Read the model definition and answer for the solid it produces. Units are mm, in the model's axes. A direction names the side the tool comes from. Round coordinates to 2 decimals unless told otherwise and drop trailing zeros. Order: outer loops, then holes, each group sorted by start corner. A loop starts at its lowest first (then second) coordinate and runs counter-clockwise, first axis right, second up. Notation, with made-up numbers: (62.25, 41) -> (69.25, 41) arc R21 ccw to (69.25, 54) -> close; hole circle Ø4 at (42.5, 82.25). An arc over 180 degrees is marked (long way). Use a Markdown table: item, result. Add a question column.
1. Section C-C, the plane z = 9 is taken. Give the vertices of the cut face in (x, y).
2. Section B-B, the plane x = -19 is taken. Give the vertices of the cut face in (y, z), then the cut area to 3 significant figures.
3. For faces 5 (the face through (-49.53, -3.94, -24.1)), 6 (the face through (48.054, -3.944, -25.806)), 7 (the face through (-1.407, -3.944, 28.093)), determine the directions among +Z, -Z, +X, -X, +Y, -Y from which every point of the face is accessible in a straight line to the end or side of a thin tool.
4. Consider L1, parallel to X at y = -3.25, z = -19; L2, parallel to X at y = -0.5, z = 22.5; L3, parallel to Z at x = -16, y = -4.25. Determine where each line is inside the solid, lowest interval first. Write a range as [from, to].
5. Given pin 1 (8 mm diameter, centred on x = -1.28, z = 22.19, fed in from +Y); pin 2 (4 mm diameter, centred on x = -27.5, y = -3.5, fed in from -Z), each flat-ended and moving along its own axis, determine where each tip first touches the part or whether it passes through.
6. Section A-A, the plane y = -4 is taken. Give the vertices of the cut face in (x, z).
7. The mould has two halves that part along X. Classify faces 1 (the face through (46.024, -3.944, -14.267)), 2 (the face through (0, 0, 2)), 3 (the face through (-31.24, -3.94, 3.5)), 4 (the face through (53.575, -3.944, -22.679)): +X half, -X half, draft (parallel to the pull), parting line (faces both ways), or undercut.
```python
from build123d import *

# Parameters (mm, degrees)
F1_DEPTH = 8
F2_R     = 2.5
F3_DEPTH = 8


# Not quite as in the source:
# - ends of sketch curves that miss each other by under 0.0002 mm in the source are joined


with BuildPart() as f1:
    # F0 (on Front) → F1 (new body)
    with BuildSketch(Plane.XZ):
        with BuildLine():
            ThreePointArc((-58.0214256358, -20.2643207275), (-54.9218439489, -24.1190997792), (-51.5609168942, -27.7482728949))
            Line((-51.5609168942, -27.7482728949), (-47.048692, -26.555894))
            ThreePointArc((-47.048692, -26.555894), (-49.5674409521, -24.0619501846), (-51.9504921504, -21.4380372685))
            Line((-51.9504921504, -21.4380372685), (-40.598231, -13.017462))
            ThreePointArc((-40.598231, -13.017462), (-0.6084110144, 0.8961956506), (40.1770750491, -10.4756859243))
            Line((40.1770750491, -10.4756859243), (52.036298, -18.165861))
            ThreePointArc((52.036298, -18.165861), (49.8229328445, -20.9344101577), (47.4659668709, -23.5817788788))
            Line((47.4659668709, -23.5817788788), (48.658346, -28.094004))
            ThreePointArc((48.658346, -28.094004), (53.6407391456, -22.5987377774), (58.0214266089, -16.6127733984))
            Line((58.0214266089, -16.6127733984), (2.355576, 26.843505))
            ThreePointArc((2.355576, 26.843505), (-1.4641584631, 28.091083381), (-5.1978982267, 26.6058182555))
            Line((-5.1978982267, 26.6058182555), (-58.0214256358, -20.2643207275))
        make_face()
    extrude(amount=F1_DEPTH)

    # F2 (on face) → F3 (cut, through all)
    with BuildSketch(Plane.XZ.offset(8)):
        with Locations((-1.27842, 22.188493)):
            Circle(F2_R)
    extrude(amount=-F3_DEPTH, mode=Mode.SUBTRACT)


solid = f1.part
```
Verdict:
| question | item | result |
|---|---|---|
| 1 | outline | (-25.04, -8) -> (25.21, -8) -> (25.21, 0) -> (-25.04, 0) -> close |
| 2 | outline | (-8, -2.14) -> (0, -2.14) -> (0, 14.36) -> (-8, 14.36) -> close |
| 2 | area | 132 mm2 |
| 3 | face 5 | +Y, -Y |
| 3 | face 6 | -Z, +Y, -Y |
| 3 | face 7 | +Z, +Y, -Y |
| 4 | L1 | x = [-56.6, -48.66], [51.39, 56.39] |
| 4 | L2 | x = [-9.83, -3.76], [1.2, 7.92] |
| 4 | L3 | z = [-1.29, 17.02] |
| 5 | pin 1 | stops at y = 0 |
| 5 | pin 2 | stops at z = -6.27 |
| 6 | outline | (-58.02, -20.26) arc R70.87 ccw to (-51.56, -27.75) -> (-47.05, -26.56) arc R66.87 cw to (-51.95, -21.44) -> (-40.6, -13.02) arc R70.87 cw to (40.18, -10.48) -> (52.04, -18.17) arc R66.87 cw to (47.47, -23.58) -> (48.66, -28.09) arc R70.87 ccw to (58.02, -16.61) -> (2.36, 26.84) arc R5.91 ccw to (-5.2, 26.61) -> close; hole circle Ø5 at (-1.28, 22.19) |
| 7 | face 1 | undercut |
| 7 | face 2 | draft |
| 7 | face 3 | -X half |
| 7 | face 4 | +X half |
